```python
from build123d import *

# Parameters (mm, degrees)
BOSS_EXTRUDE1_DEPTH = 81.28
SKETCH2_W           = 2.54
SKETCH2_H           = 16.51
CUT_REVOLVE1_ANGLE  = 180
FILLET1_R           = 1.27


with BuildPart() as part:
    # Sketch1 → Boss-Extrude1 (new body)
    with BuildSketch(Plane(origin=(0, 0, 0), x_dir=(1, 0, 0), z_dir=(0, 1, 0))):
        with BuildLine():
            Line((-68.58, 0), (-55.88, 0))
            ThreePointArc((-55.88, 0), (0, 55.88), (55.88, 0))
            Line((55.88, 0), (68.58, 0))
            ThreePointArc((68.58, 0), (0, 68.58), (-68.58, 0))
        make_face()
    extrude(amount=BOSS_EXTRUDE1_DEPTH)

    # Sketch2 → Cut-Revolve1 (revolve, cut)
    with BuildSketch(Plane.XY):
        with Locations((-67.31, 40.64)):
            Rectangle(SKETCH2_W, SKETCH2_H)
    revolve(axis=Axis((0, 81.28, 0), (0, -1, 0)), revolution_arc=CUT_REVOLVE1_ANGLE, mode=Mode.SUBTRACT)

    # Fillet1
    fillet1_edges = [part.edges().sort_by_distance(p)[0] for p in [
        (0, 48.895, -66.04),
        (0, 32.385, -66.04),
    ]]
    fillet(fillet1_edges, radius=FILLET1_R)


solid = part.part
```
Source: CAD feature listing. Evaluate the final solid. Frame: model axes, mm. A direction names the side the tool comes from. Round coordinates to 2 decimals unless told otherwise and drop trailing zeros. Loops run counter-clockwise (first coordinate to the right, second up) from the corner with the lowest first, then second, coordinate; pieces in that order, holes last. Notation, with made-up numbers: M 62,88 L 91,88 A19 ccw 91,121 Z; hole C 59,26.5 d2. An arc over 180 degrees is marked long. Use a Markdown table: item, result. Add a question column.
1. Section query A-A on x = 0. Return the cut outline in (y, z) (3 decimals), then the cut area to 3 significant figures.
2. Line query: line 1 (X direction, y = 35, z = -24.5); line 2 (X direction, y = 77, z = -41.5); line 3 (Z direction, x = 13, y = 26.5). Output: solid intervals per line, ascending.
3. Section query B-B on y = 16. Return the cut outline in (x, z), then the cut area to 3 significant figures.
4. Mould query, pull axis Y, two halves, no side actions, for faces 1 (the flat face through (0, 81.28, -57)), 2 (the flat face through (5.4, 32.385, -67.5)), 3 (the flat face through (62, 40, 0)). Classes: pulls with the +Y half, pulls with the -Y half, needs draft (parallel to the pull), parting line crosses it, or undercut.
5. Contact query for flat-ended pins moving along their axis: P1, Ø12, axis at y = 48, z = -35, coming from the +X side; P2, Ø5, axis at x = -48.5, y = 52.5, coming from the -Z side; P3, Ø4, axis at y = 29.5, z = -55.5, coming from the -X side; P4, Ø10, axis at x = 43.5, z = -16.5, coming from the -Y side. Output: stop coordinate, or through.
6. Reachability of faces 4 (the flat face through (5.4, 48.895, -67.5)), 5 (the cylindrical face through (1.508, 64.861, -68.563)) from +Z, -Z, +X, -X, +Y, -Y: full face, straight path, thin tool, end or side. Return the list, or none.
Reported:
| question | item | result |
|---|---|---|
| 1 | outline | M 0,-68.58 L 32.385,-68.58 L 32.385,-67.31 A1.27 cw 33.655,-66.04 L 47.625,-66.04 A1.27 cw 48.895,-67.31 L 48.895,-68.58 L 81.28,-68.58 L 81.28,-55.88 L 0,-55.88 Z |
| 1 | area | 991 mm² |
| 2 | line 1 | x = -61.33 to -50.22, 50.22 to 61.33 |
| 2 | line 2 | x = -54.6 to -37.42, 37.42 to 54.6 |
| 2 | line 3 | z = -67.34 to -54.35 |
| 3 | outline | M -68.58,0 A68.58 ccw 68.58,0 L 55.88,0 A55.88 cw -55.88,0 Z |
| 3 | area | 2,480 mm² |
| 4 | face 1 | pulls with the +Y half |
| 4 | face 2 | undercut |
| 4 | face 3 | needs draft |
| 5 | P1 | stops at x = 62.12 |
| 5 | P2 | stops at z = -50.86 |
| 5 | P3 | stops at x = -42.91 |
| 5 | P4 | passes through |
| 6 | face 4 | -Z |
| 6 | face 5 | -Z, +Y, -Y |
